Source: three-view drawing plus pictorial views. Frame: mm from the lowest corner of the part. Round coordinates to 2 decimals unless told otherwise and drop trailing zeros. Order: outer loops, then holes, each group sorted by start corner. A loop starts at its lowest first (then second) coordinate and runs counter-clockwise, first axis right, second up. Notation, with made-up numbers: (4.5, -3.75) -> (28.5, -3.75) arc R27 ccw to (28.5, 35.25) -> close; hole circle Ø7 at (68.25, 70.25). An arc over 180 degrees is marked (long way). Use a Markdown table: item, result.
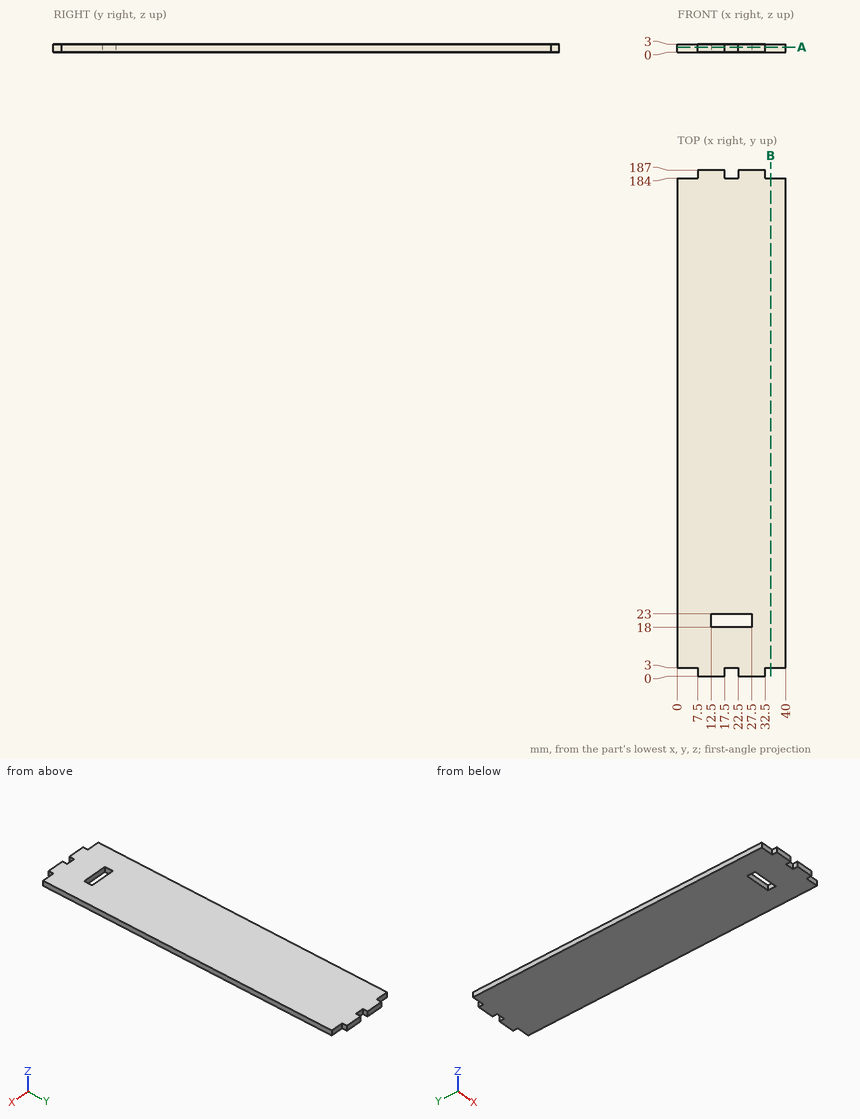
1) Pin query (flat end, axial travel): pin 1 Ø1.5 at (y, z) = (2, 2) entering from +X; pin 2 Ø1.5 at (x, z) = (4.5, 1) entering from -Y; pin 3 Ø0.9 at (x, z) = (3, 2) entering from +Y. Return the tip coordinate at first contact, or that it passes through.
Results found:
| item | result |
|---|---|
| pin 1 | stops at x = 32.5 |
| pin 2 | stops at y = 3 |
| pin 3 | stops at y = 184 |
2) Cut plane A-A on z = 1.85. Return loops of the section in (x, y), and give its area (4 significant figures).
Results found:
| item | result |
|---|---|
| outline | (0, 3) -> (7.5, 3) -> (7.5, 0) -> (17.5, 0) -> (17.5, 3) -> (22.5, 3) -> (22.5, 0) -> (32.5, 0) -> (32.5, 3) -> (40, 3) -> (40, 184) -> (32.5, 184) -> (32.5, 187) -> (22.5, 187) -> (22.5, 184) -> (17.5, 184) -> (17.5, 187) -> (7.5, 187) -> (7.5, 184) -> (0, 184) -> close; hole (12.5, 18) -> (27.5, 18) -> (27.5, 23) -> (12.5, 23) -> close |
| area | 7,285 mm² |
3) Line query: L1, parallel to Y at x = 13, z = 2.75; L2, parallel to Y at x = 21.5, z = 2.15; L3, parallel to X at y = 19, z = 1.05. Output: solid intervals per line, ascending. Write a range as [from, to].
Results found:
| item | result |
|---|---|
| L1 | y = [0, 18], [23, 187] |
| L2 | y = [3, 18], [23, 184] |
| L3 | x = [0, 12.5], [27.5, 40] |
4) Cut plane B-B on x = 34.5. Return loops of the section in (y, z), and give its area (3 significant figures).
Results found:
| item | result |
|---|---|
| outline | (3, 0) -> (184, 0) -> (184, 3) -> (3, 3) -> close |
| area | 543 mm² |
